Job drawing, mm, ordinate dimensions from the low corner. One solid piece. A direction names the side the tool comes from. Give positions to 0.01 mm unless a question says otherwise; leave off trailing zeros. Loops run counter-clockwise (first coordinate to the right, second up) from the corner with the lowest first, then second, coordinate; pieces in that order, holes last. Notation, with made-up numbers: (70.25, 26) -> (82.25, 26) arc R30 ccw to (82.25, 58) -> close; hole circle Ø5 at (45, 60.25). An arc over 180 degrees is marked (long way). Answer as a JSON object with one key per item and string values. Group by question number.
Q1. Drop flat-ended pins along their axis: pin 1 (8 mm diameter, centred on x = 28, y = 29.5, fed in from -Z); pin 2 (10 mm diameter, centred on x = 25, z = 32, fed in from -Y); pin 3 (8 mm diameter, centred on y = 23, z = 61.5, fed in from +X) (1 decimal); pin 4 (8.5 mm diameter, centred on x = 51.35, z = 51.35, fed in from -Y). Give the stop position or say it passes through.
Q2. Band-saw the part on D-D, the plane y = 31.5. Write the cut outline in (x, z) (1 decimal), plus the area to 3 significant figures.
Q3. Band-saw the part on A-A, the plane z = 50. Write the cut outline in (x, y) (1 decimal).
Q4. Band-saw the part on B-B, the plane x = 66. Write the cut outline in (y, z) (1 decimal), plus the area to 3 significant figures.
Q5. Tool access for the marked faces 1 and 2: list every direction of +Z, -Z, +X, -X, +Y, -Y with a clear straight run to the whole face (end or side of a thin tool).
Q6. Wall check: probe 1 along Y at (x, z) = (66.5, 77.5); probe 2 along X at (y, z) = (36.5, 37.5); probe 3 along Z at (x, y) = (32.5, 37) (1 decimal). Give the ranges that are in metal, low to high. Write a range as from..to.
Q7. Band-saw the part on C-C, the plane y = 12. Write the cut outline in (x, z) (1 decimal), plus the area to 3 significant figures.
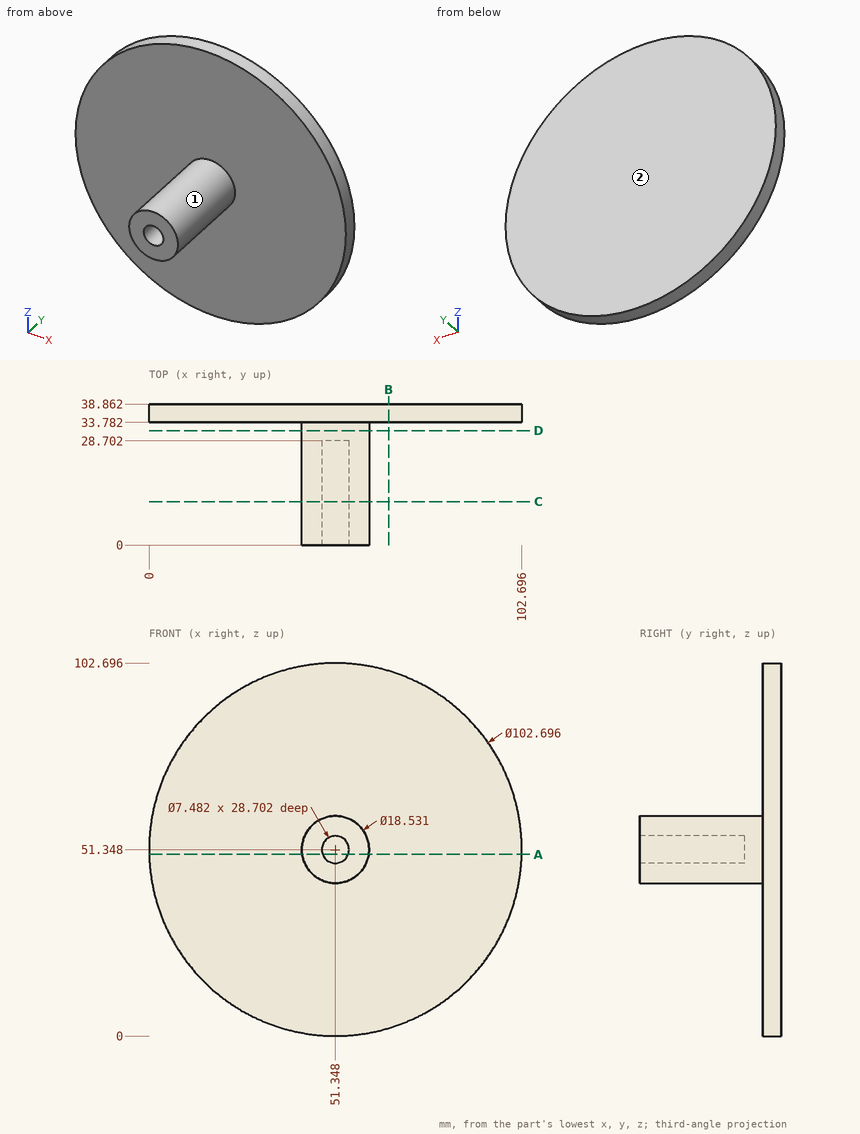
Worked answers:
{
 "1": {"pin 1": "through", "pin 2": "y = 33.78", "pin 3": "x = 58.3", "pin 4": "y = 0"},
 "2": {"outline": "circle Ø18.5 at (51.3, 51.3)", "area": "270 mm2"},
 "3": {"outline": "(0, 33.8) -> (42.2, 33.8) -> (42.2, 0) -> (47.9, 0) -> (47.9, 28.7) -> (54.8, 28.7) -> (54.8, 0) -> (60.5, 0) -> (60.5, 33.8) -> (102.7, 33.8) -> (102.7, 38.9) -> (0, 38.9) -> close"},
 "4": {"outline": "(33.8, 2.1) -> (38.9, 2.1) -> (38.9, 100.6) -> (33.8, 100.6) -> close", "area": "500 mm2"},
 "5": {"face 1": "-Y", "face 2": "+Z, -Z, +X, -X, +Y"},
 "6": {"probe 1": "33.78..38.86", "probe 2": "1.9..100.79", "probe 3": "3.6..99.1"},
 "7": {"outline": "circle Ø18.5 at (51.3, 51.3); hole circle Ø7.5 at (51.3, 51.3)", "area": "226 mm2"}
}
